Autodesk Inventor part; units mm, degrees
ref_plane "Work Plane1" through (29, 0, 0) normal (0, -1, 0) x (1, 0, 0)
ref_plane "YZ Plane" through (0, 0, 0) normal (1, 0, 0) x (0, 1, 0)
ref_plane "XZ Plane" through (0, 0, 0) normal (0, 1, 0) x (-1, 0, 0)
sketch "Sketch1" plane through (0, 0, 0) normal (0, 0, 1) x (1, 0, 0)
  line L0 (0.2709, 0) -> (9.525, 0)
  line L1 (9.525, 0) -> (9.525, 2.413)
  line L2 (9.525, 2.413) -> (2.1084, 2.413)
  line L3 (2.1084, 2.413) -> (0.0001, 2.413)
  line L4 (0.0001, 2.413) -> (0, 2.413)
  line L5 (0, 2.413) -> (0, 4.5847)
  line L6 (0, 4.5847) -> (-2.5654, 4.5847)
  line L7 (-2.5654, 4.5847) -> (-2.5654, 1.8331)
  line L8 (-2.5654, 1.8331) -> (-0.7874, 1.8331)
  line L9 (-0.7874, 1.8331) -> (0.2709, 0)
  line L10 (-4.9835, 0) -> (11.9431, 0)
  line L11 (0, -0.9169) -> (0, 5.5016)
  line L12 (2.1084, 2.413) -> (0, 2.413) construction
  dimension "d1" = 7.4166
  dimension "d2" = 2.1083
  dimension "d3" = 2.5654
  dimension "d4" = 1.778
  dimension "d5" = 60
  dimension "d6" = 4.826
  dimension "d7" = 4.826
  dimension "d8" = 3.6662
  dimension "d9" = 9.1694
  dimension "d26" = 9.525
revolve "Body" add sketch "Sketch1" angle 360 about axis through (0.2709, 0, 0) along (1, 0, 0) contours L9 L11 L3 L2 L1 L0 | L9 L8 L7 L6 L5 L11
sketch "Sketch2" plane through (-2.5654, 0, 0) normal (-1, 0, 0) x (0, 0, 1)
  circle A0 centre (0, 0) radius 1.8331
  line L0 (0, -6.4186) -> (0, 6.4186)
  line L1 (-6.4186, 0) -> (6.4186, 0)
  line L2 (1.8331, 0) -> (0.9165, -1.5875)
  line L3 (0.9165, -1.5875) -> (-0.9165, -1.5875)
  line L4 (-0.9165, -1.5875) -> (-1.8331, 0)
  line L5 (-1.8331, 0) -> (-0.9165, 1.5875)
  line L6 (-0.9165, 1.5875) -> (0.9165, 1.5875)
  line L7 (0.9165, 1.5875) -> (1.8331, 0)
  point P0 (0, 0)
extrude "Slot" add sketch "Sketch2" against normal up to next contours L7 A0 | A0 L2 | L6 L0 A0 | A0 L0 L3 | L0 L6 A0 | A0 L3 L0 | L4 A0 | A0 L5
fillet "Fillet1" radius 2.3114 1 edges at (-2.5654, -4.5847, 0)
thread "Thread"
chamfer "Chamfer1" distance 0.6492 distance2 0.6492 1 edges at (9.525, -2.413, 0) measured on face at (9.525, -0.2686, 0.7084)
ref_plane "Work Plane1" through (29, 0, 0) normal (0, -1, 0) x (1, 0, 0)
fillet "Fillet2" radius 0.1 1 edges at (0.0001, -2.413, 0)
equation "\"d1\" = GEL"
equation "\"d3\" = KOH"
equation "\"d4\" = INTI"
equation "\"d6\" = GD"
equation "\"d7\" = BDM"
equation "\"d8\" = 1.1547 * SW"
equation "\"d9\" = KOD"
equation "\"d26\" = NLG"
equation "\"d30\" = R"
equation "\"d17\" = RR"
equation "\"d13\" = GEL"
equation "\"d15\" = -0.5 * SPD + 0.5 * GD"
equation "\"d16\" = GUL"
equation "\"GD\" = NND"
equation "\"NLG\" = 9.525"
equation "\"GEL\" = 7.4166"
equation "\"KOD\" = 9.1694"
equation "\"KOH\" = 2.5654"
equation "\"INTI\" = 1.778"
equation "\"GAL\" = 2.1082"
equation "\"GUL\" = 0.64922"
equation "\"BDM\" = NND"
equation "\"SW\" = 3.175"
equation "\"RR\" = 2.3114"
equation "\"SPD\" = 3.52755"
equation "\"R\" = 0.1"
equation "\"TOA\" = 30deg"
equation "\"GD1\" = SPD"
equation "\"THREADDIA\" = 4.826"
equation "\"KOH1\" = 0.508"
equation "\"NND\" = 4.826"
equation "\"E0\" = 3.66725"
properties part number "ANSI B18.3 - 10 - 24 x 3/8" material "Steel, Mild"
Read the model definition and answer for the solid it produces. Units are mm, in the model's axes. A direction names the side the tool comes from. Give positions to 0.01 mm unless a question says otherwise; leave off trailing zeros. Order: outer loops, then holes, each group sorted by start corner. A loop starts at its lowest first (then second) coordinate and runs counter-clockwise, first axis right, second up. Notation, with made-up numbers: (78, -36.5) -> (122, -36.5) arc R35 cw to (122, -1.5) -> close; hole circle Ø3 at (4, 3.5). An arc over 180 degrees is marked (long way). Write item = value, one per line.
1. Straight lines are drawn through the part: line 1 along Z through (x, y) = (-0.25, 0); line 2 along Z through (x, y) = (-0.5, 2.75); line 3 along Z through (x, y) = (6.25, -1.5). For each, find the intervals that lie inside material, in ascending order.
Numbers:
line_1 = -4.58 to -0.9, 0.9 to 4.58
line_2 = -3.65 to 3.65
line_3 = -1.89 to 1.89
2. Given pin 1 (3 mm diameter, centred on x = 2.5, y = -3.5, fed in from +Z); pin 2 (1 mm diameter, centred on x = 0, y = -1.5, fed in from +Z); pin 3 (5 mm diameter, centred on x = 5.5, z = -1.5, fed in from -Y), each flat-ended and moving along its own axis, determine where each tip first touches the part or whether it passes through.
Numbers:
pin_1 = 1.35
pin_2 = 4.47
pin_3 = -2.41
3. The mould has two halves that part along Y. Classify faces 3 (the face through (4.427, -1.915, 1.468)), 4 (the face through (-1.62, -0.8, -1.37)), 5 (the face through (0, -1, 3)): +Y half, -Y half, draft (parallel to the pull), parting line (faces both ways), or undercut.
Numbers:
face_3 = parting line
face_4 = undercut
face_5 = draft
4. For faces 1 (the face through (-1.62, 0.8, 1.37)), 2 (the face through (-2.565, -2, 0)), determine the directions among +Z, -Z, +X, -X, +Y, -Y from which every point of the face is accessible in a straight line to the end or side of a thin tool.
Numbers:
face_1 = -X
face_2 = +Z, -Z, -X, +Y, -Y
5. A cutting plane is placed at A-A, the plane x = 8. Write down the section's boundary in (y, z).
Numbers:
outline = circle Ø4.83 at (0, 0)
